```python
from build123d import *

# Parameters (mm, degrees)
SKETCH1_R           = 1.5
BOSS_EXTRUDE1_DEPTH = 4
CHAMFER1_SIZE       = 0.15
SKETCH3_W           = 3
SKETCH3_H           = 0.8
CUT_EXTRUDE1_DEPTH  = 1


with BuildPart() as part:
    # Sketch1 → Boss-Extrude1 (new, symmetric)
    with BuildSketch(Plane.XY):
        Circle(SKETCH1_R)
    extrude(amount=BOSS_EXTRUDE1_DEPTH, both=True)

    # Chamfer1
    chamfer1_edges = [part.edges().sort_by_distance(p)[0] for p in [
        (-1.5, 0, -4),
    ]]
    chamfer(chamfer1_edges, length=CHAMFER1_SIZE)

    # Sketch3 → Cut-Extrude1 (cut)
    with BuildSketch(Plane.XY.offset(4)):
        Rectangle(SKETCH3_W, SKETCH3_H)
    extrude(amount=-CUT_EXTRUDE1_DEPTH, mode=Mode.SUBTRACT)


solid = part.part
```
The listing builds one solid part. Answer for the finished solid, in the listing's coordinates (mm). A direction names the side the tool comes from. Coordinates: 2 decimals unless noted, no trailing zeros. Loops run counter-clockwise (first coordinate to the right, second up) from the corner with the lowest first, then second, coordinate; pieces in that order, holes last. Notation, with made-up numbers: (12.25, 21.25) -> (60.25, 21.25) arc R19 cw to (60.25, 37.25) -> close; hole circle Ø7 at (52.5, -30.75). An arc over 180 degrees is marked (long way). Use one line per item in the form item = value. Start each with the question number.
Item 1: Flat-ended cylindrical pins translate along their axes: pin 1 Ø0.6 at (x, y) = (-0.5, 0) entering from +Z; pin 2 Ø1.1 at (x, z) = (0.5, 3.5) entering from -Y; pin 3 Ø1 at (x, z) = (-1, -2) entering from -Y. Find the tip coordinate at first contact, or state that the pin passes through.
Item 2: A tool of negligible diameter and unlimited length cuts with its end or side. For faces 4 (the face through (0, -1, 4)), 5 (the face through (0, -0.4, 3.5)), from which of +Z, -Z, +X, -X, +Y, -Y can it reach the whole face along a straight path? Write none if from no direction.
Item 3: The part is cut by section A-A on z = 3.25. Determine the outline of the cut face in (x, y), then the cut area to 3 significant figures.
Item 4: The part is cut by section B-B on y = 0. Determine the outline of the cut face in (x, z).
Item 5: The part is cut by section C-C on x = 0. Determine the outline of the cut face in (y, z).
Item 6: The mould has two halves that part along Y. Classify faces 1 (the face through (1.43, 0.45, 0.13)), 2 (the face through (0, 0, 3)), 3 (the face through (0, 0, -4)): released by +Y, released by -Y, zero draft, split by the parting line, or undercut.
Item 7: The part is cut by section D-D on z = -0.75. Determine the outline of the cut face in (x, y), then the cut area to 3 significant figures.
Item 8: Consider L1, parallel to Y at x = -0.65, z = -1.5; L2, parallel to Z at x = 0.45, y = 0.2; L3, parallel to Y at x = -1.2, z = -1.25. Determine where each line is inside the solid, lowest interval first. Write a range as [from, to].
Answer key:
q1.pin_1 = 3
q1.pin_2 = -1.5
q1.pin_3 = -1.41
q2.face_4 = +Z, +X, -X, +Y, -Y
q2.face_5 = +Z, +X, -X
q3.outline = (-1.45, -0.4) arc R1.5 ccw to (1.45, -0.4) -> close; (-1.45, 0.4) -> (1.45, 0.4) arc R1.5 ccw to start
q3.area = 4.70 mm2
q4.outline = (-1.5, -3.85) -> (-1.35, -4) -> (1.35, -4) -> (1.5, -3.85) -> (1.5, 3) -> (-1.5, 3) -> close
q5.outline = (-1.5, -3.85) -> (-1.35, -4) -> (1.35, -4) -> (1.5, -3.85) -> (1.5, 4) -> (0.4, 4) -> (0.4, 3) -> (-0.4, 3) -> (-0.4, 4) -> (-1.5, 4) -> close
q6.face_1 = split by the parting line
q6.face_2 = undercut
q6.face_3 = zero draft
q7.outline = circle Ø3 at (0, 0)
q7.area = 7.07 mm2
q8.L1 = [-1.35, 1.35]
q8.L2 = [-4, 3]
q8.L3 = [-0.9, 0.9]
